The figure shows three views and two pictorial views of one solid part (mm, origin at its lowest corner). Answer the questions. A direction names the side the tool comes from. Give positions to 0.01 mm unless a question says otherwise; leave off trailing zeros. Loops run counter-clockwise (first coordinate to the right, second up) from the corner with the lowest first, then second, coordinate; pieces in that order, holes last. Notation, with made-up numbers: (4.5, 34.25) - (35.5, 34.25) arc R22 ccw to (35.5, 43.25) - close; hole circle Ø3 at (-38.5, -4.75). An arc over 180 degrees is marked (long way). Use CSV: the item, a comma, the result in double quotes.
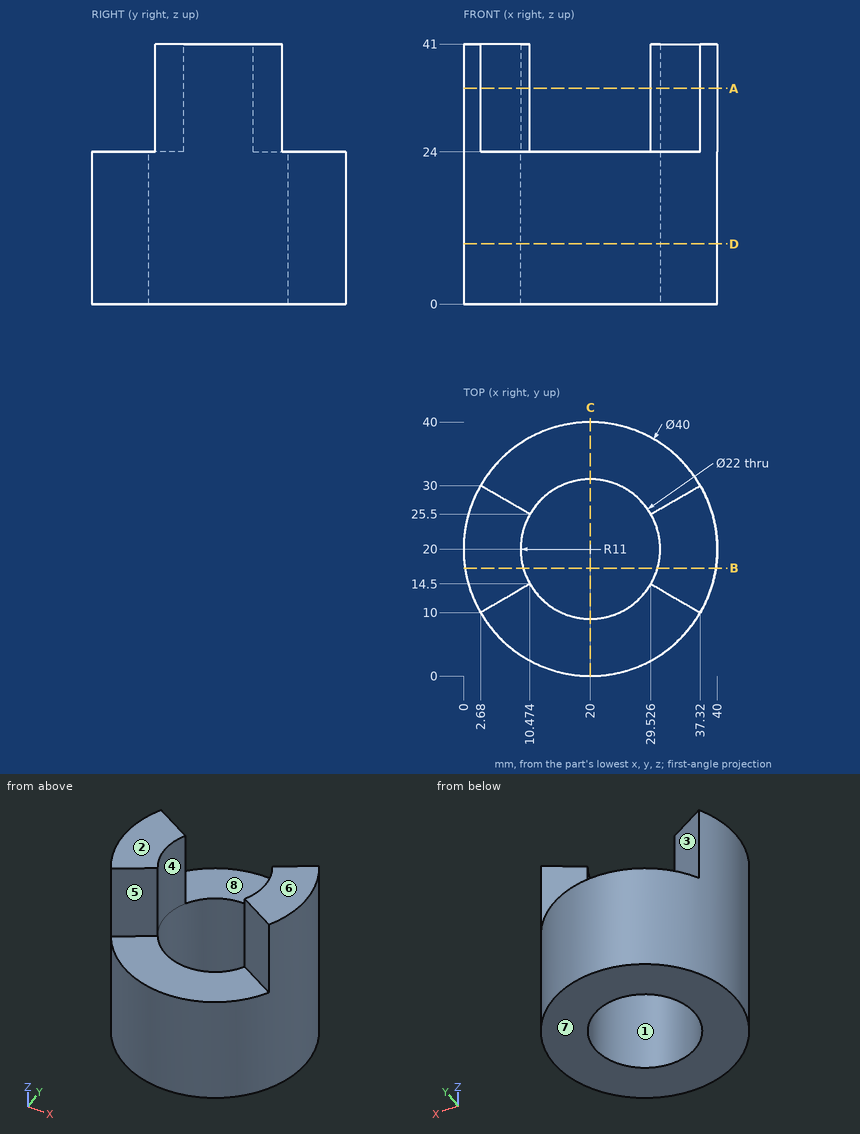
Item 1: Find the intervals of material crossed by line 1 (X direction, y = 20, z = 16); line 2 (Z direction, x = 19.5, y = 38), in increasing order.
Determined:
line 1,"x = 0 to 9, 31 to 40"
line 2,"z = 0 to 24"
Item 2: A cutting plane is placed at B-B on y = 17. Determine the outline of the cut face in (x, z).
Determined:
outline,"(0.23, 0) - (9.42, 0) - (9.42, 41) - (0.23, 41) - close; (30.58, 0) - (39.77, 0) - (39.77, 41) - (30.58, 41) - close"
Item 3: The mould has two halves that part along Y. Classify the marked faces 1, 2 and 3: pulls with the +Y half, pulls with the -Y half, needs draft (parallel to the pull), parting line crosses it, or undercut.
Determined:
face 1,"undercut"
face 2,"needs draft"
face 3,"pulls with the +Y half"
Item 4: For the marked faces 4, 5, 6, 7 and 8, determine the directions among +Z, -Z, +X, -X, +Y, -Y from which every point of the face is accessible in a straight line to the end or side of a thin tool.
Determined:
face 4,"+Z, -Z"
face 5,"+Z, -Y"
face 6,"+Z, +X, -X, +Y, -Y"
face 7,"-Z, +X, -X, +Y, -Y"
face 8,"+Z, +Y"
Item 5: A cutting plane is placed at A-A on z = 34. Determine the outline of the cut face in (x, y).
Determined:
outline,"(2.68, 10) - (10.47, 14.5) arc R11 cw to (10.47, 25.5) - (2.68, 30) arc R20 ccw to start; (29.53, 14.5) - (37.32, 10) arc R20 ccw to (37.32, 30) - (29.53, 25.5) arc R11 cw to start"
Item 6: Given P1, Ø6, axis at x = 10.5, z = 29, coming from the -Y side; P2, Ø6, axis at x = 11.5, y = 5.5, coming from the -Z side; P3, Ø11.5, axis at x = 15.5, y = 9.5, coming from the +Z side; P4, Ø8, axis at y = 25, z = 28, coming from the -X side (1 decimal), each flat-ended and moving along its own axis, determine where each tip first touches the part or whether it passes through.
Determined:
P1,"stops at y = 12.78"
P2,"stops at z = 0"
P3,"stops at z = 24"
P4,"stops at x = 0"
Item 7: A cutting plane is placed at C-C on x = 20. Determine the outline of the cut face in (y, z), and give its area (3 significant figures).
Determined:
outline,"(0, 0) - (9, 0) - (9, 24) - (0, 24) - close; (31, 0) - (40, 0) - (40, 24) - (31, 24) - close"
area,"432 mm²"
Item 8: A cutting plane is placed at D-D on z = 9.5. Determine the outline of the cut face in (x, y).
Determined:
outline,"circle Ø40 at (20, 20); hole circle Ø22 at (20, 20)"
